from build123d import *

# Parameters (mm, degrees)
PAD_DEPTH       = 10
POCKET_DEPTH    = 3.2
SKETCH002_R     = 2
POCKET001_DEPTH = 9.001


with BuildPart() as part:
    # Sketch → Pad (new body)
    with BuildSketch(Plane.XY):
        Polygon((0, 0), (0, -2.8), (4, -6.8), (11.8, -6.8), (15.8, -2.8), (15.8, 0), (11.8, 0), (11.8, 2.2), (4, 2.2), (4, 0), align=None)
    extrude(amount=PAD_DEPTH)

    # Sketch001 (on DatumPlane) → Pocket (cut)
    with BuildSketch(Plane.XZ.offset(6.8)):
        Polygon((11.5, 7.078461), (7.9, 9.156922), (4.3, 7.078461), (4.3, 2.921539), (7.9, 0.843078), (11.5, 2.921539), align=None)
    extrude(amount=-POCKET_DEPTH, mode=Mode.SUBTRACT)

    # Sketch002 (on DatumPlane) → Pocket001 (cut, through all)
    with BuildSketch(Plane.XZ.offset(6.8)):
        with Locations((7.9, 5)):
            Circle(SKETCH002_R)
    extrude(amount=-POCKET001_DEPTH, mode=Mode.SUBTRACT)


solid = part.part
Model file for the job. Use its own axes, mm. A direction names the side the tool comes from. Coordinates: 2 decimals unless noted, no trailing zeros. Write each loop counter-clockwise with the first axis right and the second up, starting at its lowest first coordinate (ties: lowest second). Pieces come first, ordered by that corner, then holes. Notation, with made-up numbers: (83, 66) -> (121, 66) arc R22 ccw to (121, 97) -> close; hole circle Ø6 at (-23, 51.25). An arc over 180 degrees is marked (long way). One line per item, written item: value. Start each with the question number.
1) Slice it at D-D on y = -3. Write the cut outline in (x, z), then the cut area to 3 significant figures.
2) Probe probe 1 along Z at (x, y) = (8, 0); probe 2 along Y at (x, z) = (10.5, 3); probe 3 along Z at (x, y) = (9, 1.5). List the from-to ranges inside material, lowest first.
3) Slice it at C-C on x = 6.25. Write the cut outline in (y, z).
4) Pull direction Z, two halves, no side cores. Call faces 1 (the face through (11.8, 1, 5)), 2 (the face through (9.675, -5.222, 1.868)), 3 (the face through (8, -2, 10)): +Z half, -Z half, draft (parallel to the pull), parting line (faces both ways), or undercut.
5) Slice it at B-B on z = 5. Write the cut outline in (x, y), then the cut area to 3 significant figures.
6) Slice it at A-A on y = -5.5. Write the cut outline in (x, z), then the cut area to 3 significant figures.
7) Which spindle directions (+Z, -Z, +X, -X, +Y, -Y) get a long thin tool onto all of the face, cutting with end or side? Do faces 4 (the face through (4, 1, 5)), 5 (the face through (6.1, -6.8, 1.6)), 6 (the face through (4.3, -5, 5)), 7 (the face through (0, -1, 5)), 8 (the face through (14, 0, 5)). Say none if no direction does.
8) Flat gauge pins, fed straight in: pin 1 Ø1.6 at (y, z) = (-5.5, 4) entering from -X; pin 2 Ø0.7 at (y, z) = (1, 3) entering from +X; pin 3 Ø3 at (x, z) = (14, 4.5) entering from +Y. Where does each tip first touch, or does it go through?
Answers follow:
1. outline: (0.2, 0) -> (15.6, 0) -> (15.6, 10) -> (0.2, 10) -> close; hole circle Ø4 at (7.9, 5)
1. area: 141 mm2
2. probe 1: 0 to 3, 7 to 10
2. probe 2: -3.6 to 2.2
2. probe 3: 0 to 3.33, 6.67 to 10
3. outline: (-6.8, 0) -> (2.2, 0) -> (2.2, 3.87) -> (-3.6, 3.87) -> (-3.6, 1.8) -> (-6.8, 1.8) -> close; (-6.8, 8.2) -> (-3.6, 8.2) -> (-3.6, 6.13) -> (2.2, 6.13) -> (2.2, 10) -> (-6.8, 10) -> close
4. face 1: draft
4. face 2: undercut
4. face 3: +Z half
5. outline: (0, -2.8) -> (4, -6.8) -> (4.3, -6.8) -> (4.3, -3.6) -> (5.9, -3.6) -> (5.9, 2.2) -> (4, 2.2) -> (4, 0) -> (0, 0) -> close; (9.9, -3.6) -> (11.5, -3.6) -> (11.5, -6.8) -> (11.8, -6.8) -> (15.8, -2.8) -> (15.8, 0) -> (11.8, 0) -> (11.8, 2.2) -> (9.9, 2.2) -> close
5. area: 62.4 mm2
6. outline: (2.7, 0) -> (13.1, 0) -> (13.1, 10) -> (2.7, 10) -> close; hole (4.3, 2.92) -> (7.9, 0.84) -> (11.5, 2.92) -> (11.5, 7.08) -> (7.9, 9.16) -> (4.3, 7.08) -> close
6. area: 59.1 mm2
7. face 4: +Z, -Z, -X, +Y
7. face 5: +Z, -Z, +X, -X, -Y
7. face 6: -Y
7. face 7: +Z, -Z, -X, +Y, -Y
7. face 8: +Z, -Z, +X, +Y
8. pin 1: x = 1.9
8. pin 2: x = 11.8
8. pin 3: y = 0
